from build123d import *

# Parameters (mm, degrees)
SKETCH1_R           = 12.512434662
BOSS_EXTRUDE1_DEPTH = 33.02
SKETCH9_W           = 25.4
SKETCH9_H           = 38.1
BOSS_EXTRUDE2_DEPTH = 3.66776
SKETCH10_W          = 76.3016
SKETCH10_H          = 31.75
BOSS_EXTRUDE3_DEPTH = 18.316200479
SKETCH13_W          = 1.467555556
SKETCH13_H          = 32.483304479
BOSS_EXTRUDE4_DEPTH = 31.75
SKETCH14_W          = 25.4635
SKETCH14_H          = 31.75
BOSS_EXTRUDE5_DEPTH = 1.467104


with BuildPart() as part:
    # Sketch1 → Boss-Extrude1 (new body)
    with BuildSketch(Plane.XY):
        Circle(SKETCH1_R)
    extrude(amount=BOSS_EXTRUDE1_DEPTH)

    # Sketch9 → Boss-Extrude2 (add)
    with BuildSketch(Plane(origin=(0, 0, 0), x_dir=(-1, 0, 0), z_dir=(0, 0, -1))):
        with Locations((0, 5.434708389)):
            Rectangle(SKETCH9_W, SKETCH9_H)
    extrude(amount=-BOSS_EXTRUDE2_DEPTH)

    # Sketch10 → Boss-Extrude3 (add)
    with BuildSketch(Plane(origin=(0, 24.484708389, 0), x_dir=(1, 0, 0), z_dir=(0, 1, 0))):
        with Locations((0, -15.875)):
            Rectangle(SKETCH10_W, SKETCH10_H)
    extrude(amount=BOSS_EXTRUDE3_DEPTH)

    # Sketch13 → Boss-Extrude4 (add)
    with BuildSketch(Plane.XY.offset(31.75)):
        with Locations((-38.884577778, 40.726360629)):
            Rectangle(SKETCH13_W, SKETCH13_H)
        with Locations((38.884577778, 40.726360629)):
            Rectangle(SKETCH13_W, SKETCH13_H)
    extrude(amount=-BOSS_EXTRUDE4_DEPTH)

    # Sketch14 → Boss-Extrude5 (add)
    with BuildSketch(Plane(origin=(0, 56.968012868, 0), x_dir=(1, 0, 0), z_dir=(0, 1, 0))):
        with Locations((-25.41905, -15.875)):
            Rectangle(SKETCH14_W, SKETCH14_H)
        with Locations((25.41905, -15.875)):
            Rectangle(SKETCH14_W, SKETCH14_H)
    extrude(amount=-BOSS_EXTRUDE5_DEPTH)


solid = part.part
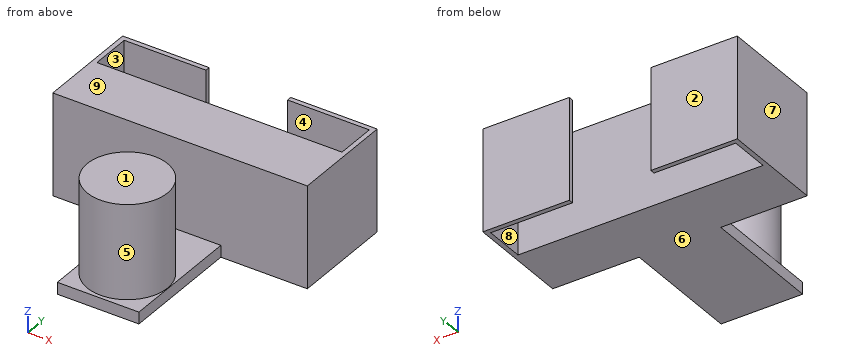
Work out the finished part from the listing and answer in its coordinate system (mm). Face numbers are marked on the shaded views. A direction names the side the tool comes from. Round coordinates to 2 decimals unless told otherwise and drop trailing zeros. Write each loop counter-clockwise with the first axis right and the second up, starting at its lowest first coordinate (ties: lowest second). Pieces come first, ordered by that corner, then holes. Notation, with made-up numbers: M 35,12.25 L 72,12.25 A24 ccw 72,22.25 Z; hole C 0.25,20.25 d6. An arc over 180 degrees is marked long. Use a Markdown table: item, result.
1) The part is cut by section D-D on x = 0. Give the vertices of the cut face in (y, z).
Taken from the geometry:
| item | result |
|---|---|
| outline | M -13.62,0 L 42.8,0 L 42.8,31.75 L 24.48,31.75 L 24.48,3.67 L 12.51,3.67 L 12.51,33.02 L -12.51,33.02 L -12.51,3.67 L -13.62,3.67 Z |
2) Which of the six approach directions +Z, -Z, +X, -X, +Y, -Y give full straight-line access (tool end or side, diameter ignored) to the marked faces 5, 6, 7, 8 and 9?
Taken from the geometry:
| item | result |
|---|---|
| face 5 | +Z |
| face 6 | -Z, +X, -X, +Y, -Y |
| face 7 | +Z, -Z, -X, +Y, -Y |
| face 8 | +Z, -Z |
| face 9 | +Z, +X, -X, +Y |
3) Determine the mould class of the marked faces 1, 2, 3 and 4 for opening direction Y: pulls with the +Y half, pulls with the -Y half, needs draft (parallel to the pull), parting line crosses it, or undercut.
Taken from the geometry:
| item | result |
|---|---|
| face 1 | needs draft |
| face 2 | pulls with the +Y half |
| face 3 | undercut |
| face 4 | undercut |
4) The part is cut by section C-C on x = -25. Give the vertices of the cut face in (y, z).
Taken from the geometry:
| item | result |
|---|---|
| outline | M 24.48,0 L 42.8,0 L 42.8,31.75 L 24.48,31.75 Z; M 55.5,0 L 56.97,0 L 56.97,31.75 L 55.5,31.75 Z |
5) The part is cut by section B-B on z = 6. Give the vertices of the cut face in (x, y), plus the area to 3 significant figures.
Taken from the geometry:
| item | result |
|---|---|
| outline | M -39.62,24.48 L 39.62,24.48 L 39.62,56.97 L 12.69,56.97 L 12.69,55.5 L 38.15,55.5 L 38.15,42.8 L -38.15,42.8 L -38.15,55.5 L -12.69,55.5 L -12.69,56.97 L -39.62,56.97 Z; C 0,0 d25.02 |
| area | 2,060 mm2 |
6) The part is cut by section A-A on y = 51. Give the vertices of the cut face in (x, z), plus the area to 3 significant figures.
Taken from the geometry:
| item | result |
|---|---|
| outline | M -39.62,0 L -38.15,0 L -38.15,31.75 L -39.62,31.75 Z; M 38.15,0 L 39.62,0 L 39.62,31.75 L 38.15,31.75 Z |
| area | 93.2 mm2 |
7) Consider line 1 (Y direction, x = 33, z = 9); line 2 (X direction, y = 49, z = 25); line 3 (Z direction, x = 14, y = 26). Determine where each line is inside the solid, lowest interval first. Write a range as [from, to].
Taken from the geometry:
| item | result |
|---|---|
| line 1 | y = [24.48, 42.8], [55.5, 56.97] |
| line 2 | x = [-39.62, -38.15], [38.15, 39.62] |
| line 3 | z = [0, 31.75] |
8) Flat-ended cylindrical pins translate along their axes: pin 1 (8 mm diameter, centred on x = -18.5, y = 17, fed in from -Z); pin 2 (1 mm diameter, centred on x = -7.5, z = 7, fed in from -Y); pin 3 (1.8 mm diameter, centred on y = 5.5, z = 2.5, fed in from -X); pin 4 (6 mm diameter, centred on x = -8.5, z = 29.5, fed in from +Y). Find the tip coordinate at first contact, or state that the pin passes through.
Taken from the geometry:
| item | result |
|---|---|
| pin 1 | passes through |
| pin 2 | stops at y = -10.37 |
| pin 3 | stops at x = -12.7 |
| pin 4 | stops at y = 42.8 |
